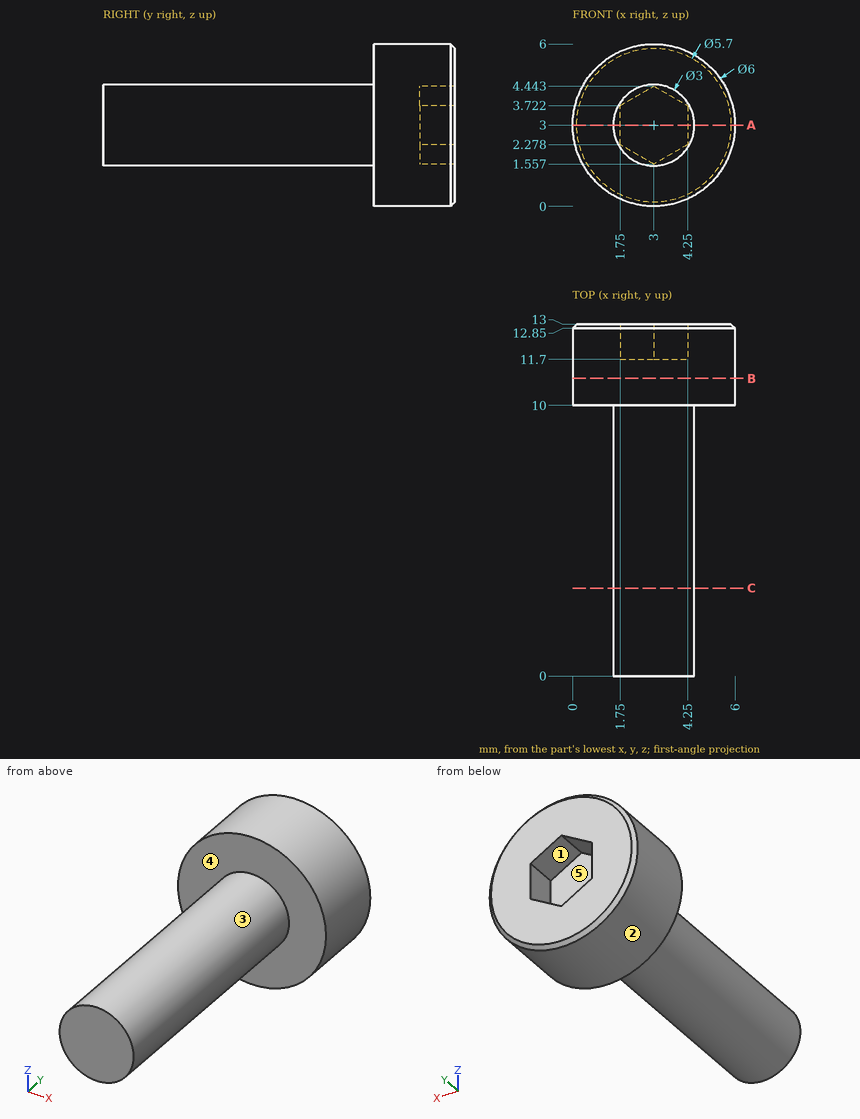
Drawing for the job (mm, zero at the part's lowest x, y, z). A direction names the side the tool comes from. Round coordinates to 2 decimals unless told otherwise and drop trailing zeros. Loops run counter-clockwise (first coordinate to the right, second up) from the corner with the lowest first, then second, coordinate; pieces in that order, holes last. Notation, with made-up numbers: M -27,16.25 L 26,16.25 A21 cw 26,29.25 Z; hole C 79,21.5 d1. An arc over 180 degrees is marked long. Use a Markdown table: item, result. Add a question column.
(1) Which spindle directions (+Z, -Z, +X, -X, +Y, -Y) get a long thin tool onto all of the face, cutting with end or side? Do the marked faces 1 and 2. Say none if no direction does.
(2) Flat gauge pins, fed straight in: pin 1 (1.5 mm diameter, centred on y = 11.5, z = 1, fed in from -X); pin 2 (3 mm diameter, centred on x = 1.5, y = 8, fed in from +Z). Where does each tip first touch, or does it go through?
(3) Drill centre lines: line 1 (Y direction, x = 2.25, z = 1); line 2 (Z direction, x = 5.6, y = 10.75) (1 decimal); line 3 (X direction, y = 11.75, z = 2.15) (1 decimal). Where is each one in solid material? Low to high.
(4) Pull direction X, two halves, no side cores. Call the marked faces 3, 4 and 5: +X half, -X half, draft (parallel to the pull), parting line (faces both ways), or undercut.
(5) Cut at A-A (z = 3). Give the cut face in (x, y).
(6) Cut at B-B (y = 11). Give the cut face in (x, z), and give its area (3 significant figures).
(7) Cut at C-C (y = 3.25). Give the cut face in (x, z).
Geometry says:
| question | item | result |
|---|---|---|
| 1 | face 1 | +Y |
| 1 | face 2 | +Y, -Y |
| 2 | pin 1 | stops at x = 0.27 |
| 2 | pin 2 | stops at z = 4.5 |
| 3 | line 1 | y = 10 to 13 |
| 3 | line 2 | z = 1.5 to 4.5 |
| 3 | line 3 | x = 0.1 to 2, 4 to 5.9 |
| 4 | face 3 | parting line |
| 4 | face 4 | draft |
| 4 | face 5 | undercut |
| 5 | outline | M 0,10 L 1.5,10 L 1.5,0 L 4.5,0 L 4.5,10 L 6,10 L 6,12.85 L 5.85,13 L 4.25,13 L 4.25,11.7 L 1.75,11.7 L 1.75,13 L 0.15,13 L 0,12.85 Z |
| 6 | outline | C 3,3 d6 |
| 6 | area | 28.3 mm² |
| 7 | outline | C 3,3 d3 |
